Read the model definition and answer for the solid it produces. Units are mm, in the model's axes. A direction names the side the tool comes from. Round coordinates to 2 decimals unless told otherwise and drop trailing zeros. Order: outer loops, then holes, each group sorted by start corner. A loop starts at its lowest first (then second) coordinate and runs counter-clockwise, first axis right, second up. Notation, with made-up numbers: (25.25, 73.5) -> (78.25, 73.5) arc R24 cw to (78.25, 99.5) -> close; hole circle Ø8 at (80.5, 18.25). An arc over 180 degrees is marked (long way). Answer as a JSON object with one key per item and string values. Group by question number.
Item 1: The mould has two halves that part along Y. Classify faces 1 (the flat face through (36.3, 20.2, -3.9)), 2 (the flat face through (39, -7, 0)), 3 (the cylindrical face through (30.74, -3.65, -3.94)): pulls with the +Y half, pulls with the -Y half, needs draft (parallel to the pull), parting line crosses it, or undercut.
Item 2: Consider probe 1 along Y at (x, z) = (78.5, -1.75); probe 2 along X at (y, z) = (-14.5, -5.75); probe 3 along Y at (x, z) = (-49, -7.5). Determine where each line is inside the solid, lowest interval first. Write a range as from..to.
Item 3: Section C-C, the plane z = -5.25 is taken. Write down the section's boundary in (x, y).
Item 4: Section B-B, the plane x = -5 is taken. Write down the section's boundary in (y, z), plus the area to 3 significant figures.
Item 5: For faces 4 (the flat face through (83, -33.5, -4)), 5 (the flat face through (-35, -16, -4)), 6 (the flat face through (99, 6.5, -4)), 7 (the flat face through (-18, -13.5, -4)), determine the directions among +Z, -Z, +X, -X, +Y, -Y from which every point of the face is accessible in a straight line to the end or side of a thin tool.
Item 6: Given P1, Ø2.5, axis at y = -15, z = -2.5, coming from the -X side; P2, Ø2, axis at x = 103.5, y = -17.5, coming from the +Z side; P3, Ø1, axis at x = 9, z = -3.5, coming from the -Y side; P4, Ø3, axis at x = -18, z = -1, coming from the -Y side, each flat-ended and moving along its own axis, determine where each tip first touches the part or whether it passes through.
Item 7: Section D-D, the plane x = 27.5 is taken. Write down the section's boundary in (y, z), plus the area to 3 significant figures.
Item 8: Section A-A, the plane y = 0 is taken. Write down the section's boundary in (x, z), plus the area to 3 significant figures.
from build123d import *

# Parameters (mm, degrees)
SKETCH_1_R             = 6
SM_BASE_FLANGE_1_DEPTH = 8


# Sheet-metal steps are written as plain solids
with BuildPart() as part:
    # Sketch 1 → Базовая кромка1 (new body)
    with BuildSketch(Plane.XY):
        with BuildLine():
            Line((-35, -13.5), (0, -13.5))
            ThreePointArc((0, -13.5), (13.5, 0), (0, 13.5))
            Line((0, 13.5), (-58.308631084, 13.5))
            Line((-58.308631084, 13.5), (-75.090623708, 33.5))
            Line((-75.090623708, 33.5), (23, 33.5))
            Line((23, 33.5), (50, 6.5))
            Line((50, 6.5), (150, 6.5))
            Line((150, 6.5), (150, -33.5))
            Line((150, -33.5), (14.5, -33.5))
            Line((14.5, -33.5), (-35, -18.5))
            Line((-35, -18.5), (-35, -13.5))
        make_face()
        with Locations((35.5, 0)):
            Circle(SKETCH_1_R, mode=Mode.SUBTRACT)
    extrude(amount=-SM_BASE_FLANGE_1_DEPTH)


solid = part.part
Values found:
{
 "1": {"face 1": "pulls with the +Y half", "face 2": "needs draft", "face 3": "undercut"},
 "2": {"probe 1": "-33.5..6.5", "probe 2": "-35..150", "probe 3": "13.5..33.5"},
 "3": {"outline": "(-75.09, 33.5) -> (-58.31, 13.5) -> (0, 13.5) arc R13.5 cw to (0, -13.5) -> (-35, -13.5) -> (-35, -18.5) -> (14.5, -33.5) -> (150, -33.5) -> (150, 6.5) -> (50, 6.5) -> (23, 33.5) -> close; hole circle Ø12 at (35.5, 0)"},
 "4": {"outline": "(-27.59, -8) -> (-13.5, -8) -> (-13.5, 0) -> (-27.59, 0) -> close; (13.5, -8) -> (33.5, -8) -> (33.5, 0) -> (13.5, 0) -> close", "area": "273 mm2"},
 "5": {"face 4": "+Z, -Z, +X, -X, -Y", "face 5": "+Z, -Z, -X, -Y", "face 6": "+Z, -Z, +X, +Y", "face 7": "+Z, -Z, -X"},
 "6": {"P1": "x = -35", "P2": "z = 0", "P3": "y = -31.98", "P4": "y = -24.11"},
 "7": {"outline": "(-33.5, -8) -> (29, -8) -> (29, 0) -> (-33.5, 0) -> close", "area": "500 mm2"},
 "8": {"outline": "(13.5, -8) -> (29.5, -8) -> (29.5, 0) -> (13.5, 0) -> close; (41.5, -8) -> (150, -8) -> (150, 0) -> (41.5, 0) -> close", "area": "996 mm2"}
}
